```python
from build123d import *

# Parameters (mm, degrees)
SKETCH1_W                 = 24.553215102
SKETCH1_H                 = 7.9375
BOSS_EXTRUDE1_DEPTH       = 18.5375
CUT_EXTRUDE2_DEPTH        = 19.5375
SKETCH3_W                 = 4.965715102
SKETCH3_H                 = 20.79375
BOSS_EXTRUDE2_DEPTH       = 8.509
CHAMFER2_SIZE             = 3.175
CHAMFER4_SIZE             = 1.27
CUT_EXTRUDE1_DEPTH        = 10.0285
HOLE1_AT_2_COUNT          = 2
HOLE1_AT_2_PITCH          = 15.553215102
HOLE1_AT_3_COUNT          = 2
HOLE1_AT_3_PITCH          = 30.296905783
HOLE1_AT_4_COUNT          = 2
HOLE1_AT_4_PITCH          = 26
F_0_CLEARANCE_HOLE1_D     = 1.8542
F_0_CLEARANCE_HOLE1_DEPTH = 6.35
F_0_CLEARANCE_HOLE1_TIP   = 0.55705788
HOLE2_AT_2_COUNT          = 2
HOLE2_AT_2_PITCH          = 15.182467652
HOLE2_AT_3_COUNT          = 2
HOLE2_AT_3_PITCH          = 29.379980379
HOLE2_AT_4_COUNT          = 2
HOLE2_AT_4_PITCH          = 33.075076063
F_0_CLEARANCE_HOLE2_D     = 1.8542
F_0_CLEARANCE_HOLE2_DEPTH = 6.35
F_0_CLEARANCE_HOLE2_TIP   = 0.55705788


with BuildPart() as part:
    # Sketch1 → Boss-Extrude1 (new body)
    with BuildSketch(Plane.XY):
        with Locations((0, -14.365625)):
            Rectangle(SKETCH1_W, SKETCH1_H)
    extrude(amount=BOSS_EXTRUDE1_DEPTH)

    # Sketch8 → Cut-Extrude2 (cut, through all)
    with BuildSketch(Plane(origin=(0, 0, 0), x_dir=(-1, 0, 0), z_dir=(0, 0, -1))):
        with BuildLine():
            Line((5.172348921, -18.334375), (12.276607551, -18.334375))
            Line((12.276607551, -18.334375), (12.276607551, -14.566653941))
            ThreePointArc((12.276607551, -14.566653941), (8.925550458, -16.829647917), (5.172348921, -18.334375))
        make_face()
        with BuildLine():
            Line((-12.276607551, -14.566653941), (-12.276607551, -18.334375))
            Line((-12.276607551, -18.334375), (-5.172348921, -18.334375))
            ThreePointArc((-5.172348921, -18.334375), (-8.925550458, -16.829647917), (-12.276607551, -14.566653941))
        make_face()
    extrude(amount=-CUT_EXTRUDE2_DEPTH, mode=Mode.SUBTRACT)


with BuildPart() as body_2:
    # Mirror2: mirrored copy
    add(part.part.mirror(Plane(origin=(0, 0, 0), x_dir=(0, 0, 1), z_dir=(0, -1, 0))))


with BuildPart() as part_1:
    add(part.part)

    add(body_2.part)  # Boss-Extrude2 merges body 2
    # Sketch3 → Boss-Extrude2 (add)
    with BuildSketch(Plane.XY.offset(18.5375)):
        Rectangle(SKETCH3_W, SKETCH3_H)
    extrude(amount=-BOSS_EXTRUDE2_DEPTH)

    # Chamfer2
    chamfer2_edges = [part_1.edges().sort_by_distance(p)[0] for p in [
        (0, 10.396875, 10.0285),
        (0, -10.396875, 10.0285),
    ]]
    chamfer(chamfer2_edges, length=CHAMFER2_SIZE)

    # Chamfer4
    chamfer4_edges = [part_1.edges().sort_by_distance(p)[0] for p in [
        (-12.276607551, -10.396875, 9.26875),
        (12.276607551, -10.396875, 9.26875),
        (-12.276607551, 10.396875, 9.26875),
        (12.276607551, 10.396875, 9.26875),
    ]]
    chamfer(chamfer4_edges, length=CHAMFER4_SIZE)

    # Sketch2 → Cut-Extrude1 (cut)
    with BuildSketch(Plane(origin=(0, 0, 0), x_dir=(-1, 0, 0), z_dir=(0, 0, -1))):
        with BuildLine():
            ThreePointArc((4.602887336, 0), (7.776607551, -11.85), (10.950327765, 0))
            ThreePointArc((10.950327765, 0), (7.776607551, 11.85), (4.602887336, 0))
        make_face()
        with BuildLine():
            ThreePointArc((-10.950327765, 0), (-7.776607551, -11.85), (-4.602887336, 0))
            ThreePointArc((-4.602887336, 0), (-7.776607551, 11.85), (-10.950327765, 0))
        make_face()
    extrude(amount=-CUT_EXTRUDE1_DEPTH, mode=Mode.SUBTRACT)

    # Sketch5 → Hole1 (revolve, cut)
    with BuildSketch(Plane(origin=(-7.776607551, 13, 18.5375), x_dir=(0, -1, 0), z_dir=(1, 0, 0))):
        Polygon((0, 0), (0, 2.921), (1.4986, 2.921), (1.6383, 0), align=None)
    hole1 = revolve(axis=Axis((-7.776607551, 13, -91.4625), (0, 0, 1)), mode=Mode.SUBTRACT)

    # Hole1 at 2: Hole1 ×2
    with Locations(*[(i * HOLE1_AT_2_PITCH, 0, 0) for i in range(1, HOLE1_AT_2_COUNT)]):
        add(hole1, mode=Mode.SUBTRACT)

    # Hole1 at 3: Hole1 ×2
    with Locations(*[Vector(0.513359853, -0.858173445, 0) * (i * HOLE1_AT_3_PITCH) for i in range(1, HOLE1_AT_3_COUNT)]):
        add(hole1, mode=Mode.SUBTRACT)

    # Hole1 at 4: Hole1 ×2
    with Locations(*[(0, -i * HOLE1_AT_4_PITCH, 0) for i in range(1, HOLE1_AT_4_COUNT)]):
        add(hole1, mode=Mode.SUBTRACT)

    # #0 Clearance Hole1
    with Locations(Plane.XY.offset(18.5375)):
        with Locations((7.776607551, 13), (7.776607551, -13), (-7.776607551, -13), (-7.776607551, 13)):
            Hole(F_0_CLEARANCE_HOLE1_D / 2, depth=F_0_CLEARANCE_HOLE1_DEPTH)
            with Locations((0, 0, -(F_0_CLEARANCE_HOLE1_DEPTH + F_0_CLEARANCE_HOLE1_TIP / 2))):  # 118° drill point
                Cone(0, F_0_CLEARANCE_HOLE1_D / 2, F_0_CLEARANCE_HOLE1_TIP, mode=Mode.SUBTRACT)

    # Sketch9 → Hole2 (revolve, cut)
    with BuildSketch(Plane(origin=(7.435045578, -14.689990189, 0), x_dir=(0, 1, 0), z_dir=(1, 0, 0))):
        Polygon((0, 0), (0, 2.921), (1.4986, 2.921), (1.6383, 0), align=None)
    hole2 = revolve(axis=Axis((7.435045578, -14.689990189, 110), (0, 0, -1)), mode=Mode.SUBTRACT)

    # Hole2 at 2: Hole2 ×2
    with Locations(*[Vector(-0.999999954, -0.000302745, 0) * (i * HOLE2_AT_2_PITCH) for i in range(1, HOLE2_AT_2_COUNT)]):
        add(hole2, mode=Mode.SUBTRACT)

    # Hole2 at 3: Hole2 ×2
    with Locations(*[(0, i * HOLE2_AT_3_PITCH, 0) for i in range(1, HOLE2_AT_3_COUNT)]):
        add(hole2, mode=Mode.SUBTRACT)

    # Hole2 at 4: Hole2 ×2
    with Locations(*[Vector(-0.459030447, 0.888420536, 0) * (i * HOLE2_AT_4_PITCH) for i in range(1, HOLE2_AT_4_COUNT)]):
        add(hole2, mode=Mode.SUBTRACT)

    # #0 Clearance Hole2
    with Locations(Plane(origin=(0, 0, 0), x_dir=(-1, 0, 0), z_dir=(0, 0, -1))):
        with Locations((-7.435045578, -14.689990189), (-7.435045578, 14.689990189), (7.747421379, 14.69458661), (7.747421379, -14.69458661)):
            Hole(F_0_CLEARANCE_HOLE2_D / 2, depth=F_0_CLEARANCE_HOLE2_DEPTH)
            with Locations((0, 0, -(F_0_CLEARANCE_HOLE2_DEPTH + F_0_CLEARANCE_HOLE2_TIP / 2))):  # 118° drill point
                Cone(0, F_0_CLEARANCE_HOLE2_D / 2, F_0_CLEARANCE_HOLE2_TIP, mode=Mode.SUBTRACT)


solid = part_1.part
```
Build history of the part. All positions in model axes, mm. A direction names the side the tool comes from. Round coordinates to 2 decimals unless told otherwise and drop trailing zeros. Loops run counter-clockwise (first coordinate to the right, second up) from the corner with the lowest first, then second, coordinate; pieces in that order, holes last.
Item 1: Which spindle directions (+Z, -Z, +X, -X, +Y, -Y) get a long thin tool onto all of the face, cutting with end or side? Do faces 4 (the face through (8.248, -14.497, 17.097)), 5 (the face through (-7.43, -11.84, 4.94)), 6 (the face through (11.77, -11.16, 9.14)), 7 (the face through (-0.03, -8.83, 8.42)), 8 (the face through (-12.277, -13, 9)). Say none if no direction does.
Item 2: Pin check, flat tips, straight feed: P1, Ø0.9, axis at x = -8.5, y = -15, coming from the -Z side; P2, Ø6, axis at y = 4, z = 13, coming from the +X side; P3, Ø5, axis at x = 6, y = 2, coming from the +Z side; P4, Ø3, axis at x = -8.5, z = 7.5, coming from the -Y side. Stop position of each tip, or through.
Item 3: Saw through at B-B (x = 0). List the corners of the cut face in (y, z), then the cut area to 3 significant figures.
Item 4: Saw through at D-D (x = 10.5). List the corners of the cut face in (y, z).
Item 5: Drill centre lines: line 1 along X through (y, z) = (13, 13.15); line 2 along Y through (x, z) = (-0.25, 5.75); line 3 along Y through (x, z) = (6.5, 17.75). Where is each one in solid material? Low to high.
Item 6: Two-plate mould, pull along Y, no slides. Class faces 1 (the face through (2.483, 0, 14)), 2 (the face through (8.875, 16.856, 9.139)), 3 (the face through (12.277, 13, 9)): released by +Y, released by -Y, zero draft, split by the parting line, or undercut.
Item 7: Saw through at A-A (z = 14). List the corners of the cut face in (x, y).
Item 8: Saw through at C-C (z = 2). List the corners of the cut face in (x, y).
Worked answers:
1. face 4: +Z
1. face 5: -Z
1. face 6: +Z, -Z, +X
1. face 7: -Z, +X, -X
1. face 8: +Z, -Z, -X, +Y, -Y
2. P1: stops at z = 2.92
2. P2: stops at x = 2.48
2. P3: passes through
2. P4: stops at y = -17.72
3. outline: (-18.33, 0) - (-10.4, 0) - (-10.4, 6.85) - (-7.22, 10.03) - (7.22, 10.03) - (10.4, 6.85) - (10.4, 0) - (18.33, 0) - (18.33, 18.54) - (-18.33, 18.54) - close
3. area: 481 mm2
4. outline: (-15.9, 0) - (-11.24, 0) - (-11.24, 10.03) - (-10.4, 10.03) - (-10.4, 18.54) - (-15.9, 18.54) - close; (10.4, 10.03) - (11.24, 10.03) - (11.24, 0) - (15.9, 0) - (15.9, 18.54) - (10.4, 18.54) - close
5. line 1: x = -12.28 to -8.7, -6.85 to 6.85, 8.7 to 12.28
5. line 2: y = -18.33 to -10.4, 10.4 to 18.33
5. line 3: y = -17.91 to -13.97, -12.03 to -10.4, 10.4 to 12.03, 13.97 to 17.91
6. face 1: undercut
6. face 2: released by +Y
6. face 3: zero draft
7. outline: (-12.28, -14.57) arc R19.05 ccw to (-5.17, -18.33) - (5.17, -18.33) arc R19.05 ccw to (12.28, -14.57) - (12.28, -11.67) - (11.01, -10.4) - (2.48, -10.4) - (2.48, 10.4) - (11.01, 10.4) - (12.28, 11.67) - (12.28, 14.57) arc R19.05 ccw to (5.17, 18.33) - (-5.17, 18.33) arc R19.05 ccw to (-12.28, 14.57) - (-12.28, 11.67) - (-11.01, 10.4) - (-2.48, 10.4) - (-2.48, -10.4) - (-11.01, -10.4) - (-12.28, -11.67) - close; hole circle Ø1.85 at (-7.78, -13); hole circle Ø1.85 at (-7.78, 13); hole circle Ø1.85 at (7.78, -13); hole circle Ø1.85 at (7.78, 13)
8. outline: (-12.28, -14.57) arc R19.05 ccw to (-5.17, -18.33) - (5.17, -18.33) arc R19.05 ccw to (12.28, -14.57) - (12.28, -11.67) - (11.36, -10.75) arc R6.35 cw to (3.73, -10.4) - (-3.73, -10.4) arc R6.35 cw to (-11.36, -10.75) - (-12.28, -11.67) - close; (-12.28, 11.67) - (-11.36, 10.75) arc R6.35 cw to (-3.73, 10.4) - (3.73, 10.4) arc R6.35 cw to (11.36, 10.75) - (12.28, 11.67) - (12.28, 14.57) arc R19.05 ccw to (5.17, 18.33) - (-5.17, 18.33) arc R19.05 ccw to (-12.28, 14.57) - close; hole circle Ø3.09 at (-7.75, -14.69); hole circle Ø3.09 at (-7.75, 14.69); hole circle Ø3.09 at (7.44, -14.69); hole circle Ø3.09 at (7.44, 14.69)
